from build123d import *

# Parameters (mm, degrees)
BOSS_EXTRUDE1_DEPTH                          = 15
SKETCH2_W                                    = 137
SKETCH2_H                                    = 26
CUT_EXTRUDE1_DEPTH                           = 7
SKETCH3_R                                    = 3
BOSS_EXTRUDE2_DEPTH                          = 142
CUT_EXTRUDE2_DEPTH                           = 35
CHAMFER1_SIZE                                = 1
FILLET1_R                                    = 1
FILLET2_R                                    = 1
CBORE_FOR_M3_HEX_SOCKET_HEAD_CAP_SCR_2_COUNT = 2
CBORE_FOR_M3_HEX_SOCKET_HEAD_CAP_SCR_2_PITCH = 17
CBORE_FOR_M3_HEX_SOCKET_HEAD_CAP_SCR_3_COUNT = 2
CBORE_FOR_M3_HEX_SOCKET_HEAD_CAP_SCR_3_PITCH = 97
CBORE_FOR_M3_HEX_SOCKET_HEAD_CAP_SCR_4_COUNT = 2
CBORE_FOR_M3_HEX_SOCKET_HEAD_CAP_SCR_4_PITCH = 98.478424033
SKETCH7_W                                    = 32
SKETCH7_H                                    = 30
BOSS_EXTRUDE3_DEPTH                          = 14
HOLE1_D                                      = 3
HOLE1_DEPTH                                  = 6


with BuildPart() as part:
    # Sketch1 → Boss-Extrude1 (new body, symmetric)
    with BuildSketch(Plane.XY):
        Polygon((-103.5, 34), (-103.5, 6), (-73.5, 6), (-73.5, 0), (73.5, 0), (73.5, 28), (68.5, 28), (68.5, 13), (-68.5, 13), (-68.5, 34), align=None)
    extrude(amount=BOSS_EXTRUDE1_DEPTH, both=True)

    # Sketch2 → Cut-Extrude1 (cut)
    with BuildSketch(Plane(origin=(0, 13, 0), x_dir=(1, 0, 0), z_dir=(0, 1, 0))):
        Rectangle(SKETCH2_W, SKETCH2_H)
    extrude(amount=-CUT_EXTRUDE1_DEPTH, mode=Mode.SUBTRACT)

    # Sketch3 → Boss-Extrude2 (add)
    with BuildSketch(Plane(origin=(73.5, 0, 0), x_dir=(0, 0, -1), z_dir=(1, 0, 0))):
        with Locations((0, 20)):
            Circle(SKETCH3_R)
    extrude(amount=-BOSS_EXTRUDE2_DEPTH)

    # Sketch4 → Cut-Extrude2 (cut, through all)
    with BuildSketch(Plane(origin=(0, 34, 0), x_dir=(1, 0, 0), z_dir=(0, 1, 0))):
        Polygon((-73.5, -15), (-73.5, -14), (-101.5, -14), (-101.5, 14), (-73.5, 14), (-73.5, 15), (-103.5, 15), (-103.5, -15), align=None)
    extrude(amount=-CUT_EXTRUDE2_DEPTH, mode=Mode.SUBTRACT)

    # Chamfer1
    chamfer1_edges = [part.edges().sort_by_distance(p)[0] for p in [
        (-87.5, 6, -14),
        (-87.5, 6, 14),
        (-87.5, 34, 14),
        (-87.5, 34, -14),
    ]]
    chamfer(chamfer1_edges, length=CHAMFER1_SIZE)

    # Fillet1
    fillet1_edges = [part.edges().sort_by_distance(p)[0] for p in [
        (-101.5, 34, 0),
        (-101.5, 20, -14),
        (-101.5, 33.5, 13.5),
        (-101.5, 33.5, -13.5),
        (-101.5, 6.5, -13.5),
        (-101.5, 6.5, 13.5),
        (-101.5, 6, 0),
        (-101.5, 20, 14),
    ]]
    fillet(fillet1_edges, radius=FILLET1_R)

    # Fillet2
    fillet2_edges = [part.edges().sort_by_distance(p)[0] for p in [
        (-71, 34, -15),
        (71, 28, -15),
        (71, 28, 15),
        (-71, 34, 15),
    ]]
    fillet(fillet2_edges, radius=FILLET2_R)

    # Sketch6 → CBORE for M3 Hex Socket Head Cap Screw1 (revolve, cut)
    with BuildSketch(Plane(origin=(-48.5, 6, -8.006829487), x_dir=(0, 0, 1), z_dir=(1, 0, 0))):
        Polygon((0, 0), (0, 6), (1.7, 6), (1.7, 3.4), (3.25, 3.4), (3.25, 0.025), (3.275, 0), align=None)
    cbore_for_m3_hex_socket_head_cap_screw1 = revolve(axis=Axis((-48.5, 12.35, -8.006829487), (0, -1, 0)), mode=Mode.SUBTRACT)

    # CBORE for M3 Hex Socket Head Cap Scr 2: CBORE for M3 Hex Socket Head Cap Screw1 ×2
    with Locations(*[(0, 0, i * CBORE_FOR_M3_HEX_SOCKET_HEAD_CAP_SCR_2_PITCH) for i in range(1, CBORE_FOR_M3_HEX_SOCKET_HEAD_CAP_SCR_2_COUNT)]):
        add(cbore_for_m3_hex_socket_head_cap_screw1, mode=Mode.SUBTRACT)

    # CBORE for M3 Hex Socket Head Cap Scr 3: CBORE for M3 Hex Socket Head Cap Screw1 ×2
    with Locations(*[(i * CBORE_FOR_M3_HEX_SOCKET_HEAD_CAP_SCR_3_PITCH, 0, 0) for i in range(1, CBORE_FOR_M3_HEX_SOCKET_HEAD_CAP_SCR_3_COUNT)]):
        add(cbore_for_m3_hex_socket_head_cap_screw1, mode=Mode.SUBTRACT)

    # CBORE for M3 Hex Socket Head Cap Scr 4: CBORE for M3 Hex Socket Head Cap Screw1 ×2
    with Locations(*[Vector(0.984987331, 0, 0.172626646) * (i * CBORE_FOR_M3_HEX_SOCKET_HEAD_CAP_SCR_4_PITCH) for i in range(1, CBORE_FOR_M3_HEX_SOCKET_HEAD_CAP_SCR_4_COUNT)]):
        add(cbore_for_m3_hex_socket_head_cap_screw1, mode=Mode.SUBTRACT)

    # Sketch7 → Boss-Extrude3 (add)
    with BuildSketch(Plane(origin=(0, 28, 0), x_dir=(1, 0, 0), z_dir=(0, 1, 0))):
        Rectangle(SKETCH7_W, SKETCH7_H)
    extrude(amount=-BOSS_EXTRUDE3_DEPTH)

    # Hole1
    with Locations(Plane(origin=(0, 28, 0), x_dir=(1, 0, 0), z_dir=(0, 1, 0))):
        with Locations((10, 10), (10, -10), (-10, -10), (-10, 10)):
            Hole(HOLE1_D / 2, depth=HOLE1_DEPTH)


solid = part.part
Input: part model. Units: mm. Frame: model coordinates. A direction names the side the tool comes from. Round coordinates to 2 decimals unless told otherwise and drop trailing zeros. Loops run counter-clockwise (first coordinate to the right, second up) from the corner with the lowest first, then second, coordinate; pieces in that order, holes last. Notation, with made-up numbers: M 4,-14 L 51,-14 A20 cw 51,14 Z; hole C 18,-3.5 d1. An arc over 180 degrees is marked long. Answer as CSV lines item,"result". Start each with the question number.
(1) Line query: line 1 (X direction, y = 17, z = 10); line 2 (Y direction, x = 3, z = -7.25); line 3 (Z direction, x = -10, y = 25). Output: solid intervals per line, ascending. Write a range as [from, to].
(2) Section B-B, the plane x = -48.5. State how many separate pieces and enclosed holes the cut face has, plus the area to 3 significant figures.
(3) Section D-D, the plane x = 36.5. Output: boundary loops of the cut face in (y, z).
(4) Reachability of faces 3 (the flat face through (-1, 10, 13)), 4 (the cylindrical face through (51.673, 4.311, -8.711)), 5 (the flat face through (-87, 20, -14)), 6 (the flat face through (71, 28, 0)) from +Z, -Z, +X, -X, +Y, -Y: full face, straight path, thin tool, end or side. Return the list, or none.
(5) First-contact query: pin 1 (1 mm diameter, centred on x = 34.5, y = 22.5, fed in from -Z); pin 2 (2 mm diameter, centred on x = 22, z = 14, fed in from +Y); pin 3 (3.5 mm diameter, centred on x = -9.5, z = 10.5, fed in from +Y); pin 4 (2 mm diameter, centred on x = 48.5, z = -8.01, fed in from -Y). Flat tips, straight axial feed; report the tip coordinate or a pass-through.
(6) Draft query along X for faces 1 (the flat face through (-1, 0, 0)), 2 (the flat face through (-16, 24, 0)). Return one class per face: released by +X, released by -X, zero draft, split by the parting line, or undercut.
(7) Section A-A, the plane x = 10. Output: boundary loops of the cut face in (y, z), plus the area to 3 significant figures.
(8) Section C-C, the plane y = 20. Output: boundary loops of the cut face in (x, z), plus the area to 3 significant figures.
Values found:
1,line 1,"x = [-101.5, -68.5], [-16, 16], [68.5, 73.5]"
1,line 2,"y = [0, 6], [14, 28]"
1,line 3,"z = [-15, -11.5], [-8.5, 8.5], [11.5, 15]"
2,separate pieces,"4"
2,enclosed holes,"0"
2,area,"174 mm²"
3,outline,"M 0,-15 L 13,-15 L 13,-13 L 6,-13 L 6,13 L 13,13 L 13,15 L 0,15 Z; C 20,0 d6"
4,face 3,"none"
4,face 4,"+Y"
4,face 5,"-Z, -X, +Y, -Y"
4,face 6,"+Z, -Z, +X, +Y"
5,pin 1,"stops at z = -2.24"
5,pin 2,"stops at y = 13"
5,pin 3,"stops at y = 28"
5,pin 4,"passes through"
6,face 1,"zero draft"
6,face 2,"undercut"
7,outline,"M 0,-15 L 13,-15 L 13,-13 L 6,-13 L 6,13 L 13,13 L 13,15 L 0,15 Z; M 14,-15 L 28,-15 L 28,-11.5 L 22,-11.5 L 22,-8.5 L 28,-8.5 L 28,8.5 L 22,8.5 L 22,11.5 L 28,11.5 L 28,15 L 14,15 Z"
7,area,"592 mm²"
8,outline,"M -101.5,-13 A1 ccw -100.5,-14 L -73.5,-14 L -73.5,-15 L -68.5,-15 L -68.5,-3 L -16,-3 L -16,-15 L 16,-15 L 16,-3 L 68.5,-3 L 68.5,-15 L 73.5,-15 L 73.5,15 L 68.5,15 L 68.5,3 L 16,3 L 16,15 L -16,15 L -16,3 L -68.5,3 L -68.5,15 L -73.5,15 L -73.5,14 L -100.5,14 A1 ccw -101.5,13 Z"
8,area,"2,670 mm²"
